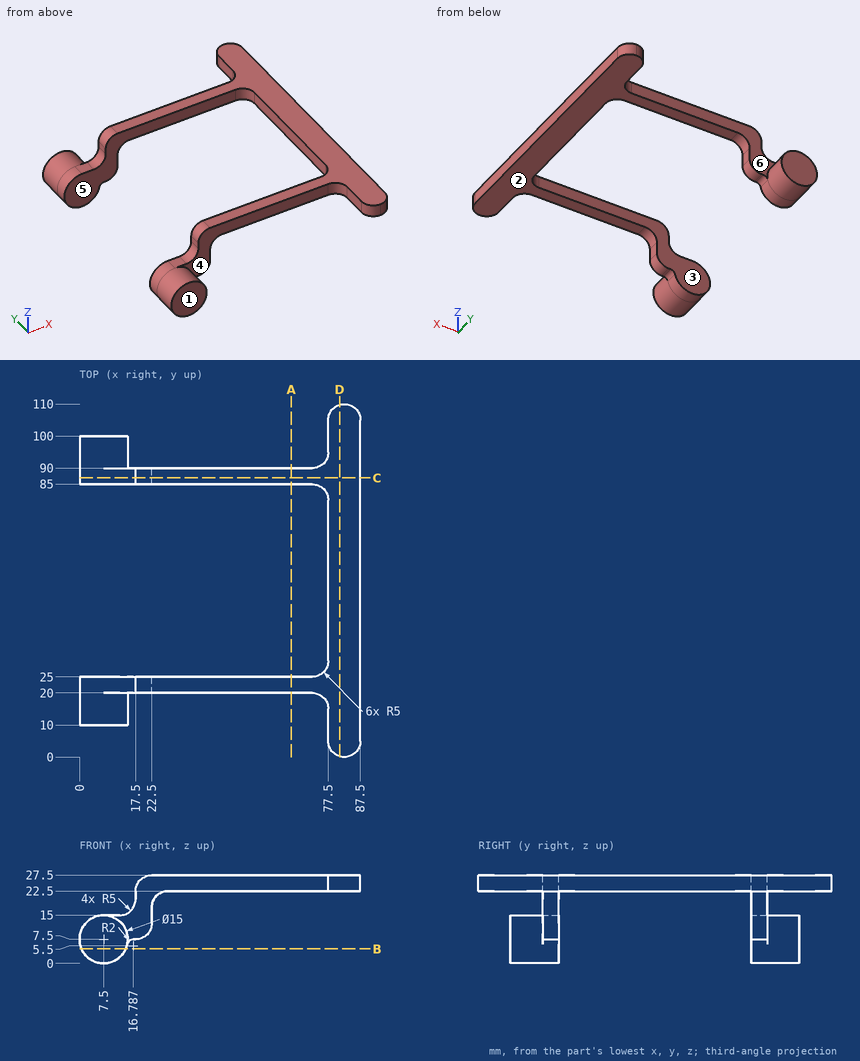
Answer from the drawing. Dimensions are ordinates in mm from the lowest x, y and z of the part. A direction names the side the tool comes from. Coordinates: 2 decimals unless noted, no trailing zeros. Loops run counter-clockwise (first coordinate to the right, second up) from the corner with the lowest first, then second, coordinate; pieces in that order, holes last. Notation, with made-up numbers: (64, 7.25) - (113, 7.25) arc R16 ccw to (113, 17.25) - close; hole circle Ø5 at (37.25, 65). An arc over 180 degrees is marked (long way). Answer in a Markdown table with one row per item.
1. Find section B-B, the plane z = 4.5. Write down the section's boundary in (x, y).
Conclusion:
| item | result |
|---|---|
| outline | (0.63, 10) - (14.37, 10) - (14.37, 25) - (0.63, 25) - close; (0.63, 85) - (14.37, 85) - (14.37, 100) - (0.63, 100) - close |
2. Straight lines are drawn through the part: line 1 (X direction, y = 71, z = 24.5); line 2 (Z direction, x = 84, y = 65); line 3 (Y direction, x = 8.5, z = 8.25). For each, find the intervals that lie inside material, in ascending order.
Conclusion:
| item | result |
|---|---|
| line 1 | x = 77.5 to 87.5 |
| line 2 | z = 22.5 to 27.5 |
| line 3 | y = 10 to 25, 85 to 100 |
3. Find section C-C, the plane y = 87. Write down the section's boundary in (x, z), then the cut area to 3 significant figures.
Conclusion:
| item | result |
|---|---|
| outline | (7.5, 15) arc R7.5 ccw (long way) to (14.83, 5.92) arc R2 cw to (16.79, 7.5) - (17.5, 7.5) arc R5 ccw to (22.5, 12.5) - (22.5, 17.5) arc R5 cw to (27.5, 22.5) - (87.5, 22.5) - (87.5, 27.5) - (22.5, 27.5) arc R5 ccw to (17.5, 22.5) - (17.5, 20) arc R5 cw to (12.5, 15) - close |
| area | 633 mm² |
4. Given pin 1 (16.5 mm diameter, centred on x = 9.5, z = 8.5, fed in from -Y); pin 2 (0.8 mm diameter, centred on x = 17, y = 88.5, fed in from -Z); pin 3 (3 mm diameter, centred on y = 23, z = 21, fed in from -X) (3 decimals), each flat-ended and moving along its own axis, determine where each tip first touches the part or whether it passes through.
Conclusion:
| item | result |
|---|---|
| pin 1 | stops at y = 10 |
| pin 2 | stops at z = 7.49 |
| pin 3 | stops at x = 17.475 |
5. Find section A-A, the plane x = 66. Write down the section's boundary in (y, z).
Conclusion:
| item | result |
|---|---|
| outline | (20, 22.5) - (25, 22.5) - (25, 27.5) - (20, 27.5) - close; (85, 22.5) - (90, 22.5) - (90, 27.5) - (85, 27.5) - close |
6. Determine the mould class of the marked faces 4, 5 and 6 for opening direction Y: +Y half, -Y half, draft (parallel to the pull), parting line (faces both ways), or undercut.
Conclusion:
| item | result |
|---|---|
| face 4 | -Y half |
| face 5 | undercut |
| face 6 | +Y half |
7. Which of the six approach directions +Z, -Z, +X, -X, +Y, -Y give full straight-line access (tool end or side, diameter ignored) to the marked faces 1, 2 and 3?
Conclusion:
| item | result |
|---|---|
| face 1 | +Z, -Z, +X, -X, -Y |
| face 2 | -Z, +X, +Y, -Y |
| face 3 | +Z, -Z, -X |
8. Find section D-D, the plane x = 81. Write down the section's boundary in (y, z), then the cut area to 3 significant figures.
Conclusion:
| item | result |
|---|---|
| outline | (0.23, 22.5) - (109.77, 22.5) - (109.77, 27.5) - (0.23, 27.5) - close |
| area | 548 mm² |
